from build123d import *

# Parameters (mm, degrees)
SKETCH1_W           = 70
SKETCH1_H           = 40
BOSS_EXTRUDE1_DEPTH = 50
SKETCH2_R           = 11
CUT_EXTRUDE1_DEPTH  = 65.226162893
SKETCH3_R           = 6
CUT_EXTRUDE2_DEPTH  = 65.226162893


with BuildPart() as part:
    # Sketch1 → Boss-Extrude1 (new body)
    with BuildSketch(Plane.XY):
        Rectangle(SKETCH1_W, SKETCH1_H)
    extrude(amount=BOSS_EXTRUDE1_DEPTH)

    # Sketch2 → Cut-Extrude1 (cut, through all)
    with BuildSketch(Plane.XY.offset(50)):
        Circle(SKETCH2_R)
    extrude(amount=-CUT_EXTRUDE1_DEPTH, mode=Mode.SUBTRACT)

    # Sketch3 → Cut-Extrude2 (cut, through all)
    with BuildSketch(Plane.XY.offset(50)):
        with Locations((-22, 0)):
            Circle(SKETCH3_R)
        with Locations((22, 0)):
            Circle(SKETCH3_R)
    extrude(amount=-CUT_EXTRUDE2_DEPTH, mode=Mode.SUBTRACT)


solid = part.part
Could you check a few things on this model? Use its own coordinates, in mm. Give positions to 0.01 mm unless a question says otherwise; leave off trailing zeros. Order: outer loops, then holes, each group sorted by start corner. A loop starts at its lowest first (then second) coordinate and runs counter-clockwise, first axis right, second up.
1. We'd pull the mould along X, two halves only. Please class faces 1 (the flat face through (35, 0, 25)), 2 (the flat face through (-35, 0, 25)), 3 (the flat face through (7, 9, 50)), 4 (the cylindrical face through (-26.76, -3.65, 25.35)): pulls with the +X half, pulls with the -X half, needs draft (parallel to the pull), parting line crosses it, or undercut.
2. Suppose I cut it at D-D (y = 9). List the corners of the cut face in (x, z) for me, plus the area to 3 significant figures.
3. Suppose I cut it at B-B (x = 0). List the corners of the cut face in (y, z) for me.
4. I need wall thicknesses on L1, parallel to Y at x = 0, z = 36; L2, parallel to Y at x = -22, z = 27.5; L3, parallel to X at y = 5, z = 38.5. Which ranges of each line are inside material? Lowest first, please.
5. Will this pin go through, and if not, where does the flat tip stop? P1, Ø9.5, axis at x = -22, y = 0, coming from the -Z side.
6. Suppose I cut it at A-A (y = 0). List the corners of the cut face in (x, z) for me.
7. Suppose I cut it at C-C (z = 41.5). List the corners of the cut face in (x, y) for me, plus the area to 3 significant figures.
Solved:
1. face 1: pulls with the +X half
1. face 2: pulls with the -X half
1. face 3: needs draft
1. face 4: undercut
2. outline: (-35, 0) - (-6.32, 0) - (-6.32, 50) - (-35, 50) - close; (6.32, 0) - (35, 0) - (35, 50) - (6.32, 50) - close
2. area: 2,870 mm2
3. outline: (-20, 0) - (-11, 0) - (-11, 50) - (-20, 50) - close; (11, 0) - (20, 0) - (20, 50) - (11, 50) - close
4. L1: y = -20 to -11, 11 to 20
4. L2: y = -20 to -6, 6 to 20
4. L3: x = -35 to -25.32, -18.68 to -9.8, 9.8 to 18.68, 25.32 to 35
5. P1: passes through
6. outline: (-35, 0) - (-28, 0) - (-28, 50) - (-35, 50) - close; (-16, 0) - (-11, 0) - (-11, 50) - (-16, 50) - close; (11, 0) - (16, 0) - (16, 50) - (11, 50) - close; (28, 0) - (35, 0) - (35, 50) - (28, 50) - close
7. outline: (-35, -20) - (35, -20) - (35, 20) - (-35, 20) - close; hole circle Ø12 at (-22, 0); hole circle Ø22 at (0, 0); hole circle Ø12 at (22, 0)
7. area: 2,190 mm2
